from build123d import *
from OCP.BRepFilletAPI import BRepFilletAPI_MakeChamfer

# Parameters (mm, degrees)
PIPESKETCH_R    = 10.668
PIPESKETCH_R_2  = 7.8994
EXTRUSION_DEPTH = 28.575
CHAMFER1_SIZE   = 0.635
CHAMFER1_SIZE2  = 0.655683131
CHAMFER2_SIZE   = 0.3175


with BuildPart() as part:
    # PipeSketch → Extrusion (new body)
    with BuildSketch(Plane.XY):
        Circle(PIPESKETCH_R)
        Circle(PIPESKETCH_R_2, mode=Mode.SUBTRACT)
    extrude(amount=EXTRUSION_DEPTH)

    # Sketch3 → Cut-Revolve1 (revolve, cut)
    with BuildSketch(Plane(origin=(0, 0, 0), x_dir=(0, 0, -1), z_dir=(1, 0, 0)), mode=Mode.PRIVATE) as cut_revolve1_sk:
        Polygon((-28.575, 10.668), (-28.575, 10.231882895), (-14.5415, 10.668), align=None)
    revolve(cut_revolve1_sk.sketch.rotate(Axis((0, 0, 0), (0, 0, 1)), 90), axis=Axis((0, 0, 0), (0, 0, 1)), mode=Mode.SUBTRACT)

    # Chamfer1: one chamfer whose edges measure the first distance from different faces: ONE call of the kernel's chamfer builder (chamfer() names one face for all edges)
    chamfer1_edges_1 = [part.edges().sort_by_distance(p)[0] for p in [
        (10.231882895, 0, 28.575),
    ]]
    chamfer1_side_1 = [part.faces().sort_by_distance(p)[0] for p in [
        (9.942481544, 0, 28.575),
    ]]
    chamfer1_edges_2 = [part.edges().sort_by_distance(p)[0] for p in [
        (-10.668, 0, 0),
    ]]
    chamfer1 = BRepFilletAPI_MakeChamfer(part.part.solid().wrapped)
    for e in chamfer1_edges_1:
        chamfer1.Add(CHAMFER1_SIZE, CHAMFER1_SIZE2, e.wrapped, chamfer1_side_1[0].wrapped)  # the first distance lies on this face
    for e in chamfer1_edges_2:
        chamfer1.Add(CHAMFER1_SIZE, e.wrapped)
    add(Compound.cast(chamfer1.Shape()), mode=Mode.REPLACE)

    # Chamfer2
    chamfer2_edges = [part.edges().sort_by_distance(p)[0] for p in [
        (-7.8994, 0, 0),
        (-7.8994, 0, 28.575),
    ]]
    chamfer(chamfer2_edges, length=CHAMFER2_SIZE)


solid = part.part
Geometry check sheet. Reference: the model listing, model coordinates, mm. Round coordinates to 2 decimals unless told otherwise and drop trailing zeros. Loops run counter-clockwise (first coordinate to the right, second up) from the corner with the lowest first, then second, coordinate; pieces in that order, holes last. Notation, with made-up numbers: (52, 56) - (57, 56) arc R15 ccw to (57, 73) - close; hole circle Ø3 at (34, 6). An arc over 180 degrees is marked (long way). Answer as CSV lines item,"result".
(1) Material ranges on line 1 along Y through (x, z) = (0, 6.25); line 2 along X through (y, z) = (-3.5, 16); line 3 along X through (y, z) = (0.5, 18.25), recorded low to high.
Output values:
line 1,"y = -10.67 to -7.9, 7.9 to 10.67"
line 2,"x = -10.03 to -7.08, 7.08 to 10.03"
line 3,"x = -10.54 to -7.88, 7.88 to 10.54"
(2) Cross-section at D-D, the plane z = 23. Enter the section's corners in (x, y), and give its area (3 significant figures).
Output values:
outline,"circle Ø20.81 at (0, 0); hole circle Ø15.8 at (0, 0)"
area,"144 mm²"
(3) Release check for a two-part mould opening along Y. For faces 1 (the face through (2.268, 10.214, 21.137)), 2 (the face through (8, 3, 28.575)), 3 (the face through (-7.89, 0.35, 14.09)) record: released by +Y, released by -Y, zero draft, split by the parting line, or undercut.
Output values:
face 1,"split by the parting line"
face 2,"zero draft"
face 3,"undercut"
(4) Cross-section at C-C, the plane z = 6. Enter the section's corners in (x, y).
Output values:
outline,"circle Ø21.34 at (0, 0); hole circle Ø15.8 at (0, 0)"
(5) Cross-section at A-A, the plane x = 0. Enter the section's corners in (y, z) (1 decimal), and give its area (3 significant figures).
Output values:
outline,"(-10.7, 0.6) - (-10, 0) - (-8.2, 0) - (-7.9, 0.3) - (-7.9, 28.3) - (-8.2, 28.6) - (-9.6, 28.6) - (-10.3, 27.9) - (-10.7, 14.5) - close; (7.9, 0.3) - (8.2, 0) - (10, 0) - (10.7, 0.6) - (10.7, 14.5) - (10.3, 27.9) - (9.6, 28.6) - (8.2, 28.6) - (7.9, 28.3) - close"
area,"151 mm²"
(6) Depth check by flat-ended pin: pin 1 Ø6 at (y, z) = (-4, 11) entering from +X; pin 2 Ø1.5 at (x, z) = (3.5, 16) entering from -Y; pin 3 Ø3 at (x, z) = (-2.5, 6) entering from -Y. Enter the tip coordinate at first touch or a pass-through.
Output values:
pin 1,"stops at x = 10.62"
pin 2,"stops at y = -10.26"
pin 3,"stops at y = -10.62"
